Build history of the part. All positions in model axes, mm. Face numbers are marked on the shaded views. Give positions to 0.01 mm unless a question says otherwise; leave off trailing zeros. Loops run counter-clockwise (first coordinate to the right, second up) from the corner with the lowest first, then second, coordinate; pieces in that order, holes last. Notation, with made-up numbers: M -27.5,-6.75 L -16.5,-6.75 A30 ccw -16.5,30.25 Z; hole C 79,-20.5 d7. An arc over 180 degrees is marked long. Put each result on its own line as item: value.
Autodesk Inventor part; units mm, degrees
ref_plane "YZ Plane" through (0, 0, 0) normal (1, 0, 0) x (0, 1, 0)
ref_plane "XZ Plane" through (0, 0, 0) normal (0, 1, 0) x (-1, 0, 0)
ref_plane "XY Plane" through (0, 0, 0) normal (0, 0, 1) x (1, 0, 0)
sketch "草圖1" plane through (0, 0, 0) normal (0, 1, 0) x (-1, 0, 0)
  line L0 (0, 0) -> (0, -11)
  line L1 (0, 0) -> (0, 11)
  line L2 (0, 11) -> (0, -11) construction
  line L3 (-3.25, 11) -> (-3.25, -11)
  line L4 (3.25, -11) -> (3.25, 11)
  arc A0 (3.25, 11) -> (-3.25, 11) centre (0, 11) ccw
  arc A1 (-3.25, -11) -> (3.25, -11) centre (0, -11) ccw
  circle A2 centre (0, 11) radius 1.5
  circle A3 centre (0, -11) radius 1.5
  dimension "d7" = 11
  dimension "d8" = 11
  dimension "d9" = 3.25
  dimension "d10" = 3
  dimension "d11" = 3
extrude "擠出1" add sketch "草圖1" along normal mid plane 3
properties part number "小零件2"
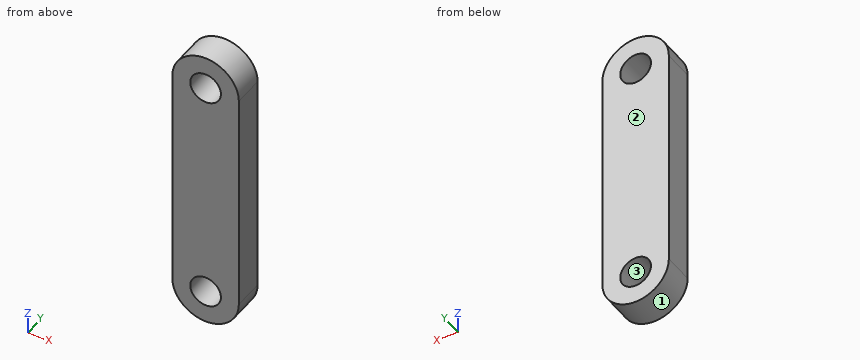
Q1. Slice it at C-C (x = 2). List the corners of the cut face in (y, z).
Here are the results:
outline: M -1.5,-13.56 L 1.5,-13.56 L 1.5,13.56 L -1.5,13.56 Z
Q2. Probe line 1 (Z direction, x = 0, y = -0.1); line 2 (X direction, y = -1.1, z = 11); line 3 (Z direction, x = 0.5, y = 0.9). List the from-to ranges inside material, lowest first. Write a range as from..to.
Here are the results:
line 1: -14.25..-12.5, -9.5..9.5, 12.5..14.25
line 2: -3.25..-1.5, 1.5..3.25
line 3: -14.21..-12.41, -9.59..9.59, 12.41..14.21
Q3. Slice it at B-B (y = -0.05). List the corners of the cut face in (x, z).
Here are the results:
outline: M -3.25,-11 A3.25 ccw 3.25,-11 L 3.25,11 A3.25 ccw -3.25,11 Z; hole C 0,-11 d3; hole C 0,11 d3
Q4. Mould opens along Z. For the marked faces 1, 2 and 3 say: pulls with the +Z half, pulls with the -Z half, needs draft (parallel to the pull), parting line crosses it, or undercut.
Here are the results:
face 1: pulls with the -Z half
face 2: needs draft
face 3: undercut
Q5. Drop a flat-ended pin along its axis: pin 1 Ø2.5 at (x, z) = (0, -11) entering from +Y. Give the stop position or say it passes through.
Here are the results:
pin 1: through
Q6. Slice it at A-A (x = 0). List the corners of the cut face in (y, z), and give its area (3 significant figures).
Here are the results:
outline: M -1.5,-14.25 L 1.5,-14.25 L 1.5,-12.5 L -1.5,-12.5 Z; M -1.5,-9.5 L 1.5,-9.5 L 1.5,9.5 L -1.5,9.5 Z; M -1.5,12.5 L 1.5,12.5 L 1.5,14.25 L -1.5,14.25 Z
area: 67.5 mm²
